Geometry: final body of the model. Coordinates: model frame, mm. Face numbers are marked on the shaded views. A direction names the side the tool comes from. Give positions to 0.01 mm unless a question says otherwise; leave off trailing zeros. Order: outer loops, then holes, each group sorted by start corner. A loop starts at its lowest first (then second) coordinate and runs counter-clockwise, first axis right, second up. Notation, with made-up numbers: (55, 61.25) - (74, 61.25) arc R27 ccw to (74, 80.25) - close; hole circle Ø10 at (60.25, 56.5). An arc over 180 degrees is marked (long way). One line per question, with ' | ' between items. Start each with the question number.
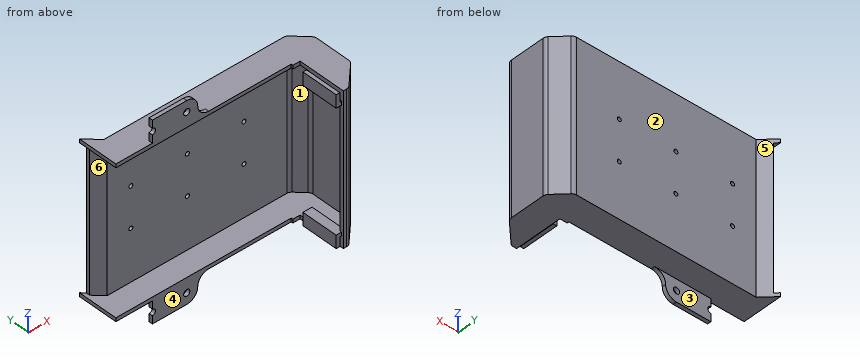
from build123d import *

# Parameters (mm, degrees)
EXTRUDE_1_DEPTH     = 82
FILLET_1_R          = 3
EXTRUDE_START       = -2
EXTRUDE_2_DEPTH     = 2
EXTRUDE_START_2     = -82
EXTRUDE_3_DEPTH     = 2
SKETCH_3_W          = 7
SKETCH_3_H          = 20
EXTRUDE_4_DEPTH     = 2
SKETCH_4_W          = 2
SKETCH_4_H          = 20
EXTRUDE_5_DEPTH     = 1
SKETCH_5_W          = 7
SKETCH_5_H          = 20
EXTRUDE_6_DEPTH     = 2
SKETCH_6_R          = 1.7
EXTRUDE_7_DEPTH     = 2
SKETCH_7_R          = 1.1
CUT_EXTRUDE_1_DEPTH = 2


with BuildPart() as part:
    # 草图1 → 凸台-拉伸1 (new body)
    with BuildSketch(Plane.XY):
        Polygon((0, 2), (3, 2), (13, 12), (13, 33.666666667), (6.666666667, 40), (-93, 40), (-98, 45), (-98, 47), (-93, 42), (6.666666667, 42), (15, 33.666666667), (15, 12), (3, 0), (0, 0), align=None)
    extrude(amount=EXTRUDE_1_DEPTH)

    # 圆角1
    fillet_1_edges = [part.edges().sort_by_distance(p)[0] for p in [
        (3, 2, 41),
        (13, 12, 41),
        (13, 33.666666667, 41),
        (6.666666667, 40, 41),
        (6.666666667, 42, 41),
        (15, 33.666666667, 41),
        (15, 12, 41),
        (3, 0, 41),
    ]]
    fillet(fillet_1_edges, radius=FILLET_1_R)

    # 草图2 → 凸台-拉伸2 (add)
    with BuildSketch(Plane(origin=(0, 0, 0), x_dir=(-1, 0, 0), z_dir=(0, 0, -1)).offset(EXTRUDE_START)):
        with BuildLine():
            Line((100, 27), (100, 49))
            Line((100, 49), (93, 42))
            Line((93, 42), (-5.42402598, 42))
            ThreePointArc((-5.42402598, 42), (-6.572076277, 41.771638598), (-7.545346323, 41.121320344))
            Line((-7.545346323, 41.121320344), (-14.121320344, 34.545346323))
            ThreePointArc((-14.121320344, 34.545346323), (-14.771638598, 33.572076277), (-15, 32.42402598))
            Line((-15, 32.42402598), (-15, 13.242640687))
            ThreePointArc((-15, 13.242640687), (-14.771638598, 12.09459039), (-14.121320344, 11.121320344))
            Line((-14.121320344, 11.121320344), (-3.878679656, 0.878679656))
            ThreePointArc((-3.878679656, 0.878679656), (-2.90540961, 0.228361402), (-1.757359313, 0))
            Line((-1.757359313, 0), (0, 0))
            Line((0, 0), (0, 26))
            Line((0, 26), (4, 26))
            Line((4, 26), (4, 27))
            Line((4, 27), (100, 27))
        make_face()
    extrude(amount=EXTRUDE_2_DEPTH)

    # 草图2<2> → 凸台-拉伸3 (add)
    with BuildSketch(Plane(origin=(0, 0, 0), x_dir=(-1, 0, 0), z_dir=(0, 0, -1)).offset(EXTRUDE_START_2)):
        with BuildLine():
            Line((100, 27), (100, 49))
            Line((100, 49), (93, 42))
            Line((93, 42), (-5.42402598, 42))
            ThreePointArc((-5.42402598, 42), (-6.572076277, 41.771638598), (-7.545346323, 41.121320344))
            Line((-7.545346323, 41.121320344), (-14.121320344, 34.545346323))
            ThreePointArc((-14.121320344, 34.545346323), (-14.771638598, 33.572076277), (-15, 32.42402598))
            Line((-15, 32.42402598), (-15, 13.242640687))
            ThreePointArc((-15, 13.242640687), (-14.771638598, 12.09459039), (-14.121320344, 11.121320344))
            Line((-14.121320344, 11.121320344), (-3.878679656, 0.878679656))
            ThreePointArc((-3.878679656, 0.878679656), (-2.90540961, 0.228361402), (-1.757359313, 0))
            Line((-1.757359313, 0), (0, 0))
            Line((0, 0), (0, 26))
            Line((0, 26), (4, 26))
            Line((4, 26), (4, 27))
            Line((4, 27), (100, 27))
        make_face()
    extrude(amount=EXTRUDE_3_DEPTH)

    # 草图3 → 凸台-拉伸4 (add)
    with BuildSketch(Plane.ZY):
        with Locations((4.5, 11)):
            Rectangle(SKETCH_3_W, SKETCH_3_H)
        with Locations((77.5, 11)):
            Rectangle(SKETCH_3_W, SKETCH_3_H)
    extrude(amount=-EXTRUDE_4_DEPTH)

    # 草图4 → 凸台-拉伸5 (add)
    with BuildSketch(Plane.ZY):
        with Locations((7, 11)):
            Rectangle(SKETCH_4_W, SKETCH_4_H)
        with Locations((75, 11)):
            Rectangle(SKETCH_4_W, SKETCH_4_H)
    extrude(amount=EXTRUDE_5_DEPTH)

    # 草图5 → 凸台-拉伸6 (add)
    with BuildSketch(Plane.ZY.offset(1)):
        with Locations((4.5, 11)):
            Rectangle(SKETCH_5_W, SKETCH_5_H)
        with Locations((77.5, 11)):
            Rectangle(SKETCH_5_W, SKETCH_5_H)
    extrude(amount=EXTRUDE_6_DEPTH)

    # 草图6 → 凸台-拉伸7 (add)
    # profile 1 of 2: a face of its own
    with BuildSketch(Plane.XZ.offset(-27)):
        with BuildLine():
            Line((-80, 86.3), (-80, 82))
            Line((-80, 82), (-49.173938425, 82))
            ThreePointArc((-49.173938425, 82), (-53.416579112, 83.757359313), (-55.173938425, 88))
            ThreePointArc((-55.173938425, 88), (-56.931297738, 92.242640687), (-61.173938425, 94))
            Line((-61.173938425, 94), (-80, 94))
            Line((-80, 94), (-80, 89.7))
            ThreePointArc((-80, 89.7), (-78.3, 88), (-80, 86.3))
        make_face()
        with Locations((-61.173938425, 88)):
            Circle(SKETCH_6_R, mode=Mode.SUBTRACT)
    # profile 2 of 2: a face of its own
    with BuildSketch(Plane.XZ.offset(-27)):
        with BuildLine():
            Line((-80, -12), (-61.173938425, -12))
            ThreePointArc((-61.173938425, -12), (-56.931297738, -10.242640687), (-55.173938425, -6))
            ThreePointArc((-55.173938425, -6), (-53.416579112, -1.757359313), (-49.173938425, 0))
            Line((-49.173938425, 0), (-80, 0))
            Line((-80, 0), (-80, -4.3))
            ThreePointArc((-80, -4.3), (-78.3, -6), (-80, -7.7))
            Line((-80, -7.7), (-80, -12))
        make_face()
        with Locations(Location((-61.173938425, -6, 0), (0, 0, 180))):
            Circle(SKETCH_6_R, mode=Mode.SUBTRACT)
    extrude(amount=-EXTRUDE_7_DEPTH)

    # 草图7 → 切除-拉伸1 (cut)
    with BuildSketch(Plane(origin=(0, 42, 0), x_dir=(1, 0, 0), z_dir=(0, 1, 0))):
        with Locations(Location((-49, -30, 0), (0, 0, 270))):
            Circle(SKETCH_7_R)
        with Locations(Location((-80, -30, 0), (0, 0, 270))):
            Circle(SKETCH_7_R)
        with Locations(Location((-80, -52, 0), (0, 0, 90))):
            Circle(SKETCH_7_R)
        with Locations(Location((-49, -52, 0), (0, 0, 90))):
            Circle(SKETCH_7_R)
        with Locations(Location((-18, -30, 0), (0, 0, 270))):
            Circle(SKETCH_7_R)
        with Locations(Location((-18, -52, 0), (0, 0, 270))):
            Circle(SKETCH_7_R)
    extrude(amount=-CUT_EXTRUDE_1_DEPTH, mode=Mode.SUBTRACT)


solid = part.part
(1) Pull-direction query (Z, two-part tool) for the marked faces 1 and 2; classes: +Z half, -Z half, draft (parallel to the pull), parting line (faces both ways), or undercut.
(2) Material intervals for line 1 along Z through (x, y) = (-87, 37.5); line 2 along X through (y, z) = (41, 30); line 3 along X through (y, z) = (40.75, 30), sorted ascending. Write a range as from..to.
(3) Cut plane C-C, the plane z = 37. Return the cut outline in (x, y).
(4) Cut plane D-D, the plane y = 5. Return the cut outline in (x, z).
(5) Access query for the marked faces 3, 4, 5 and 6. Directions: +Z, -Z, +X, -X, +Y, -Y. A direction counts if a zero-diameter tool reaches every point of the face in a straight line with its end or side. Return the directions, or none.
(6) Cut plane B-B, the plane y = 30.5. Return the cut outline in (x, z).
(7) Cut plane A-A, the plane x = -29. Return the cut outline in (y, z), plus the area to 3 significant figures.
(8) Contact query for flat-ended pins moving along their axis: P1, Ø2.5, axis at x = -61.17, z = 88, coming from the +Y side; P2, Ø8, axis at y = 39, z = 25.5, coming from the +X side; P3, Ø14.5, axis at x = -37.5, y = 21.5, coming from the +Z side; P4, Ø1, axis at x = -2, y = 7, coming from the +Z side. Output: stop coordinate, or through.
Results are:
1) face 1: undercut | face 2: draft
2) line 1: 0..2, 80..82 | line 2: -94..-81.1, -78.9..-50.1, -47.9..-19.1, -16.9..7.67 | line 3: -93.75..-81.1, -78.9..-50.1, -47.9..-19.1, -16.9..7.92
3) outline: (-98, 45) - (-93, 40) - (5.42, 40) arc R3 cw to (7.55, 39.12) - (12.12, 34.55) arc R3 cw to (13, 32.42) - (13, 13.24) arc R3 cw to (12.12, 11.12) - (3.88, 2.88) arc R3 cw to (1.76, 2) - (0, 2) - (0, 0) - (1.76, 0) arc R3 ccw to (3.88, 0.88) - (14.12, 11.12) arc R3 ccw to (15, 13.24) - (15, 32.42) arc R3 ccw to (14.12, 34.55) - (7.55, 41.12) arc R3 ccw to (5.42, 42) - (-93, 42) - (-98, 47) - close
4) outline: (-3, 1) - (-1, 1) - (-1, 6) - (0, 6) - (0, 0) - (8, 0) - (8, 82) - (0, 82) - (0, 76) - (-1, 76) - (-1, 81) - (-3, 81) - (-3, 74) - (2, 74) - (2, 80) - (6, 80) - (6, 2) - (2, 2) - (2, 8) - (-3, 8) - close
5) face 3: -Z, +X, -X, +Y | face 4: +Z, -Z, -X, -Y | face 5: +Z, -Z, +X, +Y | face 6: -X, -Y
6) outline: (-100, 0) - (15, 0) - (15, 82) - (-100, 82) - (-100, 80) - (13, 80) - (13, 2) - (-100, 2) - close
7) outline: (27, 0) - (42, 0) - (42, 82) - (27, 82) - (27, 80) - (40, 80) - (40, 2) - (27, 2) - close | area: 216 mm2
8) P1: through | P2: x = 13.67 | P3: z = 82 | P4: z = 81
